from build123d import *

# Parameters (mm, degrees)
F0_W = 40
F0_H = 12.7


with BuildPart() as f1:
    # F0 (on Front) → F1 (revolve)
    with BuildSketch(Plane.XZ):
        Polygon((-622, 0), (-622, 63.5), (-662, 63.5), (-662, 50.8), (-662, 12.7), (-662, 0), align=None)
    revolve(axis=Axis((0, 0, 31.75), (0, 0, -1)))

    # F0 (on Front) → F2 (revolve)
    with BuildSketch(Plane.XZ):
        Polygon((-662, 50.8), (-662, 63.5), (-712, 63.5), (-712, 50.8), (-672, 50.8), align=None)
        with Locations((-692, 44.45)):
            Rectangle(F0_W, F0_H)
    revolve(axis=Axis((0, 0, 31.75), (0, 0, -1)))

    # F0 (on Front) → F3 (revolve)
    with BuildSketch(Plane.XZ):
        with Locations((-692, 19.05)):
            Rectangle(F0_W, F0_H)
        Polygon((-712, 0), (-662, 0), (-662, 12.7), (-672, 12.7), (-712, 12.7), align=None)
    revolve(axis=Axis((0, 0, 31.75), (0, 0, -1)))


solid = f1.part
Work out the finished part from the listing and answer in its coordinate system (mm). A direction names the side the tool comes from. Round coordinates to 2 decimals unless told otherwise and drop trailing zeros. Loops run counter-clockwise (first coordinate to the right, second up) from the corner with the lowest first, then second, coordinate; pieces in that order, holes last. Notation, with made-up numbers: (47, 20.25) - (91, 20.25) arc R10 ccw to (91, 26.25) - close; hole circle Ø1 at (-22, 7.5). An arc over 180 degrees is marked (long way). Use one line per item in the form item = value. Start each with the question number.
(1) Consider line 1 (Y direction, x = 0, z = 16); line 2 (X direction, y = -235, z = 45.5); line 3 (Y direction, x = 378, z = 48). Determine where each line is inside the solid, lowest interval first.
(2) Find section A-A on x = 0. Determine the outline of the cut face in (y, z).
(3) Determine the mould class of faces 1 (the face through (-640.97, 201.85, 44.54)), 2 (the face through (-3, -630, 63.5)), 3 (the face through (524.774, 481.203, 12.522)) for opening direction X: +X half, -X half, draft (parallel to the pull), parting line (faces both ways), or undercut.
(4) Find section B-B on y = 47.5. Determine the outline of the cut face in (x, z).
(5) Which of the six approach directions +Z, -Z, +X, -X, +Y, -Y give full straight-line access (tool end or side, diameter ignored) to faces 4 (the face through (524.774, 481.203, 50.622)), 5 (the face through (-524, 425, 25.4))?
(6) Flat-ended cylindrical pins translate along their axes: P1, Ø2, axis at x = 52, z = 54, coming from the +Y side; P2, Ø6, axis at y = -415.5, z = 32, coming from the -X side; P3, Ø1.5, axis at y = -529.5, z = 40, coming from the -X side. Find the tip coordinate at first contact, or state that the pin passes through.
Answer list:
q1.line_1 = -712 to -672, -662 to -622, 622 to 662, 672 to 712
q1.line_2 = -672.1 to -629.57, -618.89 to -575.9, 575.9 to 618.89, 629.57 to 672.1
q1.line_3 = -603.37 to -555.61, -543.47 to -493.96, 493.96 to 543.47, 555.61 to 603.37
q2.outline = (-712, 0) - (-622, 0) - (-622, 63.5) - (-712, 63.5) - (-712, 38.1) - (-672, 38.1) - (-672, 50.8) - (-662, 50.8) - (-662, 12.7) - (-672, 12.7) - (-672, 25.4) - (-712, 25.4) - close; (622, 0) - (712, 0) - (712, 25.4) - (672, 25.4) - (672, 12.7) - (662, 12.7) - (662, 50.8) - (672, 50.8) - (672, 38.1) - (712, 38.1) - (712, 63.5) - (622, 63.5) - close
q3.face_1 = undercut
q3.face_2 = draft
q3.face_3 = parting line
q4.outline = (-710.41, 0) - (-620.18, 0) - (-620.18, 63.5) - (-710.41, 63.5) - (-710.41, 38.1) - (-670.32, 38.1) - (-670.32, 50.8) - (-660.29, 50.8) - (-660.29, 12.7) - (-670.32, 12.7) - (-670.32, 25.4) - (-710.41, 25.4) - close; (620.18, 0) - (710.41, 0) - (710.41, 25.4) - (670.32, 25.4) - (670.32, 12.7) - (660.29, 12.7) - (660.29, 50.8) - (670.32, 50.8) - (670.32, 38.1) - (710.41, 38.1) - (710.41, 63.5) - (620.18, 63.5) - close
q5.face_4 = +Z, -Z
q5.face_5 = none
q6.P1 = 710.17
q6.P2 = -517.77
q6.P3 = -476.83
